from build123d import *

# Parameters (mm, degrees)
SKETCH001_R   = 7
SKETCH001_R_2 = 19.05
PAD_DEPTH     = 15.875


with BuildPart() as part:
    # Sketch → Revolution (revolve)
    with BuildSketch(Plane.XZ):
        Polygon((19.05, 0), (19.05, 51.2064), (25.4, 51.2064), (25.4, 36.068), (43.4, 36.068), (51.05, 0), align=None)
    revolve(axis=Axis((0, 0, 0), (0, 0, 1)))

    # Sketch001 → Pad (new body)
    with BuildSketch(Plane.XY):
        with BuildLine():
            ThreePointArc((-51.005, 65.0875), (-60.962831, 60.962831), (-65.0875, 51.005))
            Line((-65.0875, -51.005), (-65.0875, 51.005))
            ThreePointArc((-65.0875, -51.005), (-60.962831, -60.962831), (-51.005, -65.0875))
            Line((51.005, -65.0875), (-51.005, -65.0875))
            ThreePointArc((51.005, -65.0875), (60.962831, -60.962831), (65.0875, -51.005))
            Line((65.0875, 51.005), (65.0875, -51.005))
            ThreePointArc((65.0875, 51.005), (60.962831, 60.962831), (51.005, 65.0875))
            Line((-51.005, 65.0875), (51.005, 65.0875))
        make_face()
        with Locations((51.005, 51.005)):
            Circle(SKETCH001_R, mode=Mode.SUBTRACT)
        with Locations((-51.005, 51.005)):
            Circle(SKETCH001_R, mode=Mode.SUBTRACT)
        with Locations((-51.005, -51.005)):
            Circle(SKETCH001_R, mode=Mode.SUBTRACT)
        with Locations((51.005, -51.005)):
            Circle(SKETCH001_R, mode=Mode.SUBTRACT)
        Circle(SKETCH001_R_2, mode=Mode.SUBTRACT)
    extrude(amount=PAD_DEPTH)


solid = part.part
Could you check a few things on this model? Use its own coordinates, in mm. A direction names the side the tool comes from. Coordinates: 2 decimals unless noted, no trailing zeros. Write each loop counter-clockwise with the first axis right and the second up, starting at its lowest first coordinate (ties: lowest second). Pieces come first, ordered by that corner, then holes. Notation, with made-up numbers: (19.25, 23) - (76.25, 23) arc R11 ccw to (76.25, 37) - close; hole circle Ø3 at (68.5, 29.5). An arc over 180 degrees is marked (long way). Put each result on its own line as item: value. Start each with the question number.
Q1. I'm going to push flat-ended pins straight in: P1, Ø3, axis at y = 28, z = 23.5, coming from the +X side; P2, Ø8, axis at x = 37.5, y = -2.5, coming from the -Z side; P3, Ø18, axis at x = -51.005, y = -51.005, coming from the +Z side (3 decimals). Where does each tip first touch, or does it pass through?
Q2. Thinking about a two-plate mould opening in X: for faces 1 (the flat face through (-65.088, -1, 8)), 2 (the cylindrical face through (-56.56, -55.264, 7.826)), 3 (the cylindrical face through (-58, 51.3, 7.8)), 4 (the flat face through (1, -65.088, 8)), which applies, pulls with the +X half, pulls with the -X half, needs draft (parallel to the pull), parting line crosses it, or undercut?
Q3. I want a section at C-C on z = 10.5. Count the separate pieces of the cut face and the enclosed holes in it, plus the area to 3 significant figures.
Q4. I want a section at D-D on z = 41. Write out the boundary of the cut face in (x, y).
Q5. Please list where these lines run through material, in increasing order: L1, parallel to X at y = -47, z = 5; L2, parallel to Z at x = 54, y = -1 (3 decimals); L3, parallel to Y at x = 8, z = 31.5.
Q6. Which directions (+Z, -Z, +X, -X, +Y, -Y) give clear straight access to the entire face, cutting with the end or side of a thin tool? Please do faces 5 (the flat face through (-19, -19, 36.068)), 6 (the cylindrical face through (60.853, -61.072, 7.826)).
Checks:
1. P1: x = 37.75
1. P2: z = 0
1. P3: z = 15.875
2. face 1: pulls with the -X half
2. face 2: undercut
2. face 3: undercut
2. face 4: needs draft
3. separate pieces: 1
3. enclosed holes: 5
3. area: 15,000 mm²
4. outline: circle Ø50.8 at (0, 0); hole circle Ø38.1 at (0, 0)
5. L1: -65.09 to -56.75, -45.26 to 45.26, 56.75 to 65.09
5. L2: 0 to 15.875
5. L3: -43.64 to -17.29, 17.29 to 43.64
6. face 5: +Z
6. face 6: +Z, -Z, +X, -Y
